```python
from build123d import *

# Parameters (mm, degrees)
SKETCH1_R           = 1.6
SKETCH1_R_2         = 5
BOSS_EXTRUDE1_DEPTH = 3


with BuildPart() as part:
    # Sketch1 → Boss-Extrude1 (new body)
    with BuildSketch(Plane(origin=(0, 0, 0), x_dir=(1, 0, 0), z_dir=(0, 1, 0))):
        with BuildLine():
            Line((-9.9, 27.5), (-9.9, -6.192201576))
            ThreePointArc((-9.9, -6.192201576), (-7.485730167, -10.104724514), (-2.905997097, -9.701512952))
            Line((-2.905997097, -9.701512952), (5.93857688, -3.001078121))
            ThreePointArc((5.93857688, -3.001078121), (8.855047984, 0.519324784), (9.9, 4.96984336))
            Line((9.9, 4.96984336), (9.9, 27.5))
            ThreePointArc((9.9, 27.5), (8.435533906, 31.035533906), (4.9, 32.5))
            Line((4.9, 32.5), (-4.9, 32.5))
            ThreePointArc((-4.9, 32.5), (-8.435533906, 31.035533906), (-9.9, 27.5))
        make_face()
        with Locations((-4.95, 7.5)):
            Circle(SKETCH1_R, mode=Mode.SUBTRACT)
        with Locations((-4.95, -7.5)):
            Circle(SKETCH1_R, mode=Mode.SUBTRACT)
        with Locations((4.95, 0)):
            Circle(SKETCH1_R, mode=Mode.SUBTRACT)
        with Locations((0, 22.5)):
            Circle(SKETCH1_R_2, mode=Mode.SUBTRACT)
    extrude(amount=BOSS_EXTRUDE1_DEPTH)


solid = part.part
```
Read the model definition and answer for the solid it produces. Units are mm, in the model's axes. Coordinates: 2 decimals unless noted, no trailing zeros. Order: outer loops, then holes, each group sorted by start corner. A loop starts at its lowest first (then second) coordinate and runs counter-clockwise, first axis right, second up. Notation, with made-up numbers: (51, 7) - (102, 7) arc R35 ccw to (102, 46) - close; hole circle Ø8 at (-27.5, 34). An arc over 180 degrees is marked (long way). Answer as a JSON object with one key per item and string values. Group by question number.
Item 1: The mould has two halves that part along X. Classify faces 1 (the face through (-7.55, 1.48, 10.07)), 2 (the face through (-9.9, 1, -11)), 3 (the face through (-4.21, 1.48, -6.08)): +X half, -X half, draft (parallel to the pull), parting line (faces both ways), or undercut.
Item 2: Consider probe 1 along X at (y, z) = (1.9, -22.5); probe 2 along Z at (x, y) = (4.5, 0.3); probe 3 along Z at (x, y) = (4.25, 0.2). Determine where each line is inside the solid, lowest interval first. Write a range as from..to.
Item 3: Section A-A (x = 0) is taken. Give the vertices of the cut face in (y, z).
Item 4: Flat-ended cylindrical pins translate along their axes: P1, Ø1.5, axis at x = 1, z = -6, coming from the -Y side; P2, Ø1, axis at x = 1, y = 2.5, coming from the +Z side. Find the tip coordinate at first contact, or state that the pin passes through.
Item 5: Section B-B (y = 2.5) is taken. Give the vertices of the cut face in (x, z), plus the area to 3 significant figures.
Item 6: Section D-D (x = -4.25) is taken. Give the vertices of the cut face in (y, z), plus the area to 3 significant figures.
Item 7: Section C-C (z = 8.5) is taken. Give the vertices of the cut face in (x, y).
Results are:
{
 "1": {"face 1": "parting line", "face 2": "-X half", "face 3": "undercut"},
 "2": {"probe 1": "x = -9.9..-5, 5..9.9", "probe 2": "z = -32.5..-24.68, -20.32..-1.54, 1.54..4.09", "probe 3": "z = -32.5..-25.13, -19.87..-1.44, 1.44..4.28"},
 "3": {"outline": "(0, -32.5) - (3, -32.5) - (3, -27.5) - (0, -27.5) - close; (0, -17.5) - (3, -17.5) - (3, 7.5) - (0, 7.5) - close"},
 "4": {"P1": "stops at y = 0", "P2": "stops at z = 7.12"},
 "5": {"outline": "(-9.9, -27.5) arc R5 ccw to (-4.9, -32.5) - (4.9, -32.5) arc R5 ccw to (9.9, -27.5) - (9.9, -4.97) arc R10 ccw to (5.94, 3) - (-2.91, 9.7) arc R4.38 ccw to (-9.9, 6.19) - close; hole circle Ø3.2 at (-4.95, -7.5); hole circle Ø3.2 at (-4.95, 7.5); hole circle Ø10 at (0, -22.5); hole circle Ø3.2 at (4.95, 0)", "area": "658 mm^2"},
 "6": {"outline": "(0, -32.5) - (3, -32.5) - (3, -25.13) - (0, -25.13) - close; (0, -19.87) - (3, -19.87) - (3, -8.94) - (0, -8.94) - close; (0, -6.06) - (3, -6.06) - (3, 6.06) - (0, 6.06) - close; (0, 8.94) - (3, 8.94) - (3, 10.38) - (0, 10.38) - close", "area": "95.6 mm^2"},
 "7": {"outline": "(-9.24, 0) - (-6.2, 0) - (-6.2, 3) - (-9.24, 3) - close; (-3.7, 0) - (-1.32, 0) - (-1.32, 3) - (-3.7, 3) - close"}
}
